Check sheet for the modelled part. Datum: model origin and axes. Units: mm. A direction names the side the tool comes from. Round coordinates to 2 decimals unless told otherwise and drop trailing zeros. Order: outer loops, then holes, each group sorted by start corner. A loop starts at its lowest first (then second) coordinate and runs counter-clockwise, first axis right, second up. Notation, with made-up numbers: M 76,52 L 108,52 A27 cw 108,75 Z; hole C 6,-31 d3. An arc over 180 degrees is marked long. One line per item, written item: value. Start each with the question number.
(1) Access from +Z, -Z, +X, -X, +Y, -Y to the whole of each face (thin tool, end or side, straight path). Record for faces 4 (the face through (51.33, -4.2, -1.6)), 5 (the face through (34.7, -6.4, -3.25)), 6 (the face through (-43, 3, 9.25)), 7 (the face through (30, 1.501, 3)), 8 (the face through (-49, 0, 3)).
(2) Depth check by flat-ended pin: pin 1 Ø4 at (x, y) = (14, -4) entering from -Z; pin 2 Ø5 at (y, z) = (5.5, 4.5) entering from +X; pin 3 Ø6 at (y, z) = (-10.5, 6.5) entering from +X. Enter the tip coordinate at first touch or a pass-through.
(3) Cross-section at A-A, the plane z = -1.75. Enter the section's corners in (x, y), and give its area (3 significant figures).
(4) Cross-section at D-D, the plane y = 0. Count the separate pieces of the cut face and the enclosed holes in it, and give its area (3 significant figures).
(5) Release check for a two-part mould opening along Y. For faces 1 (the face through (30, -1.499, 3)), 2 (the face through (51.942, 1.273, 5.588)), 3 (the face through (-43, -3, -3.25)) record: released by +Y, released by -Y, zero draft, split by the parting line, or undercut.
(6) Thickness scan on L1, parallel to X at y = 0, z = 2; L2, parallel to Y at x = -38, z = 4; L3, parallel to Y at x = 38, z = -2.05. Record the ranges inside material, lowest first.
(7) Cross-section at B-B, the plane z = 3.75. Enter the section's corners in (x, y), and give its area (3 significant figures).
from build123d import *

# Parameters (mm, degrees)
F0_R     = 5.5
F1_DEPTH = 6
F4_DEPTH = 3.25
F2_R     = 13.9763796755
F5_DEPTH = 3.25
F3_R     = 5.5
F6_DEPTH = 3.25
F7_R     = 5.5
F8_DEPTH = 3.25


with BuildPart() as f1:
    # F0 (on Top) → F1 (new body)
    with BuildSketch(Plane.XY):
        with BuildLine():
            ThreePointArc((27.8112338211, -13.6084181209), (21, 0), (27.8112338211, 13.6084181209))
            Line((27.8112338211, 13.6084181209), (-29.7807062004, 11.3332788475))
            ThreePointArc((-29.7807062004, 11.3332788475), (-24, 0), (-29.7807062004, -11.3332788475))
            Line((-29.7807062004, -11.3332788475), (27.8112338211, -13.6084181209))
        make_face()
        with BuildLine():
            ThreePointArc((-29.7807062004, -11.3332788475), (-24, 0), (-29.7807062004, 11.3332788475))
            Line((-29.7807062004, 11.3332788475), (-38.4342105263, 10.9914267144))
            ThreePointArc((-38.4342105263, 10.9914267144), (-30.3768876366, 7.9302054131), (-27, 0))
            ThreePointArc((-27, 0), (-30.3768876366, -7.9302054131), (-38.4342105263, -10.9914267144))
            Line((-38.4342105263, -10.9914267144), (-29.7807062004, -11.3332788475))
        make_face()
        with BuildLine():
            ThreePointArc((-27, 0), (-30.3768876366, 7.9302054131), (-38.4342105263, 10.9914267144))
            ThreePointArc((-38.4342105263, 10.9914267144), (-49, 0), (-38.4342105263, -10.9914267144))
            ThreePointArc((-38.4342105263, -10.9914267144), (-30.3768876366, -7.9302054131), (-27, 0))
        make_face()
        with Locations((-38, 0)):
            Circle(F0_R, mode=Mode.SUBTRACT)
        with BuildLine():
            ThreePointArc((37.4473684211, -13.9890885456), (24, 0), (37.4473684211, 13.9890885456))
            Line((37.4473684211, 13.9890885456), (27.8112338211, 13.6084181209))
            ThreePointArc((27.8112338211, 13.6084181209), (21, 0), (27.8112338211, -13.6084181209))
            Line((27.8112338211, -13.6084181209), (37.4473684211, -13.9890885456))
        make_face()
        with BuildLine():
            ThreePointArc((37.4473684211, -13.9890885456), (47.702143008, -10.0929887076), (52, 0))
            ThreePointArc((52, 0), (47.702143008, 10.0929887076), (37.4473684211, 13.9890885456))
            ThreePointArc((37.4473684211, 13.9890885456), (24, 0), (37.4473684211, -13.9890885456))
        make_face()
        with BuildLine():
            ThreePointArc((31.1628594053, 1.5011690405), (44.9999998977, -0.0011968644), (31.1623464634, -1.4988309156))
            Line((31.1623464634, -1.4988309156), (28.1623464634, -1.4988309156))
            Line((28.1623464634, -1.4988309156), (28.1628594053, 1.5011690405))
            Line((28.1628594053, 1.5011690405), (31.1628594053, 1.5011690405))
        make_face(mode=Mode.SUBTRACT)
    extrude(amount=F1_DEPTH)

    # F3 (on face) → F4 (join)
    with BuildSketch(Plane.XY.offset(6)):
        with BuildLine():
            ThreePointArc((52, 0), (47.702143008, 10.0929887076), (37.4473684211, 13.9890885456))
            ThreePointArc((37.4473684211, 13.9890885456), (24, 0), (37.4473684211, -13.9890885456))
            ThreePointArc((37.4473684211, -13.9890885456), (47.702143008, -10.0929887076), (52, 0))
        make_face()
        with BuildLine():
            Line((31.1623464634, -1.4988309156), (28.1623464634, -1.4988309156))
            Line((28.1623464634, -1.4988309156), (28.1628594053, 1.5011690405))
            Line((28.1628594053, 1.5011690405), (31.1628594053, 1.5011690405))
            ThreePointArc((31.1628594053, 1.5011690405), (44.9999998977, -0.0011968644), (31.1623464634, -1.4988309156))
        make_face(mode=Mode.SUBTRACT)
    extrude(amount=F4_DEPTH)

    # F2 (on face) → F5 (join)
    with BuildSketch(Plane(origin=(0, 0, 0), x_dir=(1, 0, 0), z_dir=(0, 0, -1))):
        with Locations((38, 0)):
            Circle(F2_R)
        with BuildLine():
            Line((28.1623464634, 1.4988309156), (31.1623464634, 1.4988309156))
            ThreePointArc((31.1623464634, 1.4988309156), (44.9999998977, 0.0011968644), (31.1628594053, -1.5011690405))
            Line((31.1628594053, -1.5011690405), (28.1628594053, -1.5011690405))
            Line((28.1628594053, -1.5011690405), (28.1623464634, 1.4988309156))
        make_face(mode=Mode.SUBTRACT)
    extrude(amount=F5_DEPTH)

    # F3 (on face) → F6 (join)
    with BuildSketch(Plane.XY.offset(6)):
        with BuildLine():
            ThreePointArc((-38.4342105263, -10.9914267144), (-30.3768876366, -7.9302054131), (-27, 0))
            ThreePointArc((-27, 0), (-30.3768876366, 7.9302054131), (-38.4342105263, 10.9914267144))
            ThreePointArc((-38.4342105263, 10.9914267144), (-49, 0), (-38.4342105263, -10.9914267144))
        make_face()
        with Locations((-38, 0)):
            Circle(F3_R, mode=Mode.SUBTRACT)
    extrude(amount=F6_DEPTH)

    # F7 (on face) → F8 (join)
    with BuildSketch(Plane(origin=(0, 0, 0), x_dir=(1, 0, 0), z_dir=(0, 0, -1))):
        with BuildLine():
            ThreePointArc((-38.4342105263, -10.9914267144), (-30.3768876366, -7.9302054131), (-27, 0))
            ThreePointArc((-27, 0), (-30.3768876366, 7.9302054131), (-38.4342105263, 10.9914267144))
            ThreePointArc((-38.4342105263, 10.9914267144), (-49, 0), (-38.4342105263, -10.9914267144))
        make_face()
        with Locations((-38, 0)):
            Circle(F7_R, mode=Mode.SUBTRACT)
    extrude(amount=F8_DEPTH)


solid = f1.part
Values found:
1. face 4: -Z
1. face 5: -Z, +X, -X, +Y, -Y
1. face 6: +Z, +X, -X, +Y, -Y
1. face 7: +Z, -Z
1. face 8: none
2. pin 1: z = 0
2. pin 2: x = 51.67
2. pin 3: x = 49.82
3. outline: C -38,0 d22; C 38,0 d27.95; hole C -38,0 d11; hole M 28.16,-1.5 L 31.16,-1.5 A7 ccw long 31.16,1.5 L 28.16,1.5 Z
3. area: 736 mm^2
4. separate pieces: 3
4. enclosed holes: 0
4. area: 583 mm^2
5. face 1: undercut
5. face 2: split by the parting line
5. face 3: zero draft
6. L1: -49 to -43.5, -32.5 to 28.16, 45 to 52
6. L2: -11.01 to -5.5, 5.5 to 11.01
6. L3: -13.98 to -7, 7 to 13.98
7. outline: M -38.43,-10.99 L 37.45,-13.99 A14 ccw long 37.45,13.99 L -38.43,10.99 A11 ccw Z; hole C -38,0 d11; hole M 28.16,-1.5 L 31.16,-1.5 A7 ccw long 31.16,1.5 L 28.16,1.5 Z
7. area: 2,140 mm^2
